```python
from build123d import *

# Parameters (mm, degrees)
SKETCH047_R          = 1.75
SKETCH047_R_2        = 1.3375
PAD025_DEPTH         = 6.5
POCKET021_DEPTH      = 25.001
POCKET021_DEPTH_BACK = 25.001
SKETCH056_W          = 1
SKETCH056_H          = 22.95
SKETCH056_H_2        = 7
POCKET025_DEPTH      = 1


with BuildPart() as part:
    # Sketch047 → Pad025 (new body)
    with BuildSketch(Plane.YZ):
        Polygon((-10, 30.95), (10, 30.95), (10, 15.95), (25, 9), (25, 0), (-25, 0), (-25, 9), (-10, 15.95), align=None)
        with Locations((-7.5, 28.45)):
            Circle(SKETCH047_R, mode=Mode.SUBTRACT)
        with Locations((7.5, 28.45)):
            Circle(SKETCH047_R, mode=Mode.SUBTRACT)
        with Locations((7.5, 18.45)):
            Circle(SKETCH047_R, mode=Mode.SUBTRACT)
        with Locations((-7.5, 18.45)):
            Circle(SKETCH047_R, mode=Mode.SUBTRACT)
        with Locations((-20, 4.5)):
            Circle(SKETCH047_R_2, mode=Mode.SUBTRACT)
        with Locations((0, 4.5)):
            Circle(SKETCH047_R_2, mode=Mode.SUBTRACT)
        with Locations((20, 4.5)):
            Circle(SKETCH047_R_2, mode=Mode.SUBTRACT)
    extrude(amount=PAD025_DEPTH)

    # Sketch048 → Pocket021 (cut, two sides)
    with BuildSketch(Plane.XZ) as pocket021_sk:
        Polygon((0, 15.95), (0, 0), (1, 0), (1, 9), align=None)
    extrude(amount=-POCKET021_DEPTH, mode=Mode.SUBTRACT)
    extrude(pocket021_sk.sketch, amount=POCKET021_DEPTH_BACK, mode=Mode.SUBTRACT)

    # Sketch056 (on Face4 of Pocket021) → Pocket025 (cut)
    with BuildSketch(Plane(origin=(0, 0, 0), x_dir=(0, 1, 0), z_dir=(-1, 0, 0))):
        with Locations((0, -11.475)):
            Rectangle(SKETCH056_W, SKETCH056_H)
        with Locations((0, -27.45)):
            Rectangle(SKETCH056_W, SKETCH056_H_2)
        with Locations((-2, -11.475)):
            Rectangle(SKETCH056_W, SKETCH056_H)
        with Locations((-2, -27.45)):
            Rectangle(SKETCH056_W, SKETCH056_H_2)
        with Locations((2, -11.475)):
            Rectangle(SKETCH056_W, SKETCH056_H)
        with Locations((2, -27.45)):
            Rectangle(SKETCH056_W, SKETCH056_H_2)
    extrude(amount=-POCKET025_DEPTH, mode=Mode.SUBTRACT)


with BuildPart() as part_1:
    # Body011 placement: moved
    add(part.part.moved(Location((-141.5, -20, 60.5))))


solid = part_1.part
```
The listing builds one solid part. Answer for the finished solid, in the listing's coordinates (mm). A direction names the side the tool comes from. Coordinates: 2 decimals unless noted, no trailing zeros. Order: outer loops, then holes, each group sorted by start corner. A loop starts at its lowest first (then second) coordinate and runs counter-clockwise, first axis right, second up. Notation, with made-up numbers: M 87.5,89.25 L 99.5,89.25 A19 ccw 99.5,122.25 Z; hole C 2.25,14 d8. An arc over 180 degrees is marked long. Answer as a JSON object with one key per item and string values. Group by question number.
1. Section B-B on z = 88.95 is taken. Write down the section's boundary in (x, y).
2. Section A-A on y = -27.5 is taken. Write down the section's boundary in (x, z), then the cut area to 3 significant figures.
3. Straight lines are drawn through the part: line 1 (Y direction, x = -139.5, z = 78.95); line 2 (Z direction, x = -136.5, y = -12.5); line 3 (Y direction, x = -139.2, z = 65). For each, find the intervals that lie inside material, in ascending order.
4. Section D-D on y = -20 is taken. Write down the section's boundary in (x, z).
5. Flat-ended cylindrical pins translate along their axes: P1, Ø0.5, axis at x = -141, z = 75, coming from the -Y side; P2, Ø1.1, axis at x = -141, z = 88.5, coming from the +Y side; P3, Ø0.8, axis at x = -141, z = 77, coming from the -Y side. Find the tip coordinate at first contact, or state that the pin passes through.
6. Section C-C on x = -137.5 is taken. State how many separate pieces and enclosed holes the cut face has, then the cut area to 3 significant figures.
7. Determine the mould class of faces 4 (the flat face through (-138.3, -2.6, 73.02)), 5 (the cylindrical face through (-138.3, -27.88, 77.24)), 6 (the flat face through (-138.3, -37.6, 72.93)), 7 (the flat face through (-138, -20, 91.45)) for opening direction Y: released by +Y, released by -Y, zero draft, split by the parting line, or undercut.
8. A tool of negligible diameter and unlimited length cuts with its end or side. For faces 1 (the flat face through (-141, -21.5, 78)), 2 (the flat face through (-141, -18.5, 88)), 3 (the flat face through (-140.88, -31.09, 72.15)), from which of +Z, -Z, +X, -X, +Y, -Y can it reach the whole face along a straight path? Write none if from no direction.
Values follow:
{
 "1": {"outline": "M -141.5,-30 L -135,-30 L -135,-29.25 L -141.5,-29.25 Z; M -141.5,-25.75 L -135,-25.75 L -135,-14.25 L -141.5,-14.25 L -141.5,-17.5 L -140.5,-17.5 L -140.5,-18.5 L -141.5,-18.5 L -141.5,-19.5 L -140.5,-19.5 L -140.5,-20.5 L -141.5,-20.5 L -141.5,-21.5 L -140.5,-21.5 L -140.5,-22.5 L -141.5,-22.5 Z; M -141.5,-10.75 L -135,-10.75 L -135,-10 L -141.5,-10 Z"},
 "2": {"outline": "M -141.5,76.45 L -140.5,69.5 L -140.5,60.5 L -135,60.5 L -135,77.2 L -141.5,77.2 Z; M -141.5,80.7 L -135,80.7 L -135,87.2 L -141.5,87.2 Z; M -141.5,90.7 L -135,90.7 L -135,91.45 L -141.5,91.45 Z", "area": "143 mm2"},
 "3": {"line 1": "-30 to -29.25, -25.75 to -14.25, -10.75 to -10", "line 2": "60.5 to 77.2, 80.7 to 87.2, 90.7 to 91.45", "line 3": "-45 to -41.34, -38.66 to -21.34, -18.66 to -1.34, 1.34 to 5"},
 "4": {"outline": "M -141.5,83.45 L -140.5,83.45 L -140.5,66.34 L -135,66.34 L -135,91.45 L -140.5,91.45 L -140.5,84.45 L -141.5,84.45 Z; M -140.5,60.5 L -135,60.5 L -135,63.66 L -140.5,63.66 Z"},
 "5": {"P1": "y = -33.67", "P2": "y = -10", "P3": "y = -30"},
 "6": {"separate pieces": "1", "enclosed holes": "7", "area": "938 mm2"},
 "7": {"face 4": "released by +Y", "face 5": "undercut", "face 6": "released by -Y", "face 7": "zero draft"},
 "8": {"face 1": "-Z, -X", "face 2": "+Z, -X", "face 3": "-Z, -X, +Y, -Y"}
}
